from build123d import *

# Parameters (mm, degrees)
SKETCH002_R     = 2.2
SKETCH002_R_2   = 1.45
PAD002_DEPTH    = 15.5
SKETCH003_R     = 33
SKETCH003_R_2   = 2.2
PAD003_DEPTH    = 4.5
POCKET_DEPTH    = 3
POCKET001_DEPTH = 4
POCKET003_DEPTH = 2
SKETCH011_W     = 5.5
SKETCH011_H     = 11.1
POCKET004_DEPTH = 25.001
SKETCH012_W     = 3.4
SKETCH012_H     = 17.1165875376
PAD007_DEPTH    = 7.75
POCKET005_DEPTH = 229.0145930205
SKETCH017_R     = 0.75
POCKET008_DEPTH = 17.1165875376
PAD008_DEPTH    = 5
SKETCH020_R     = 0.75
POCKET009_DEPTH = 1.3324822377
FILLET_R        = 0.5
FILLET001_R     = 0.5
FILLET002_R     = 3


with BuildPart() as part:
    # Sketch002 (on Face1 of ShapeBinder) → Pad002 (new body)
    with BuildSketch(Plane.XZ.offset(37.5)):
        with BuildLine():
            Line((-32.0156211872, -8), (32.0156211872, -8))
            ThreePointArc((26.9599822671, -19.0304849165), (29.9991391555, -13.7496054463), (32.0156211872, -8))
            Line((-26.9599822671, -19.0304849165), (26.9599822671, -19.0304849165))
            ThreePointArc((-32.0156211872, -8), (-29.9991391555, -13.7496054463), (-26.9599822671, -19.0304849165))
        make_face()
        with Locations((24, -11)):
            Circle(SKETCH002_R, mode=Mode.SUBTRACT)
        with Locations((0, -11)):
            Circle(SKETCH002_R_2, mode=Mode.SUBTRACT)
        with Locations((-24, -11)):
            Circle(SKETCH002_R, mode=Mode.SUBTRACT)
    extrude(amount=PAD002_DEPTH)

    # Sketch003 (on Face9 of Pad002) → Pad003 (join)
    with BuildSketch(Plane.XZ.offset(53)):
        Circle(SKETCH003_R)
        with Locations((24, -11)):
            Circle(SKETCH003_R_2, mode=Mode.SUBTRACT)
        with Locations((-24, -11)):
            Circle(SKETCH003_R_2, mode=Mode.SUBTRACT)
    extrude(amount=PAD003_DEPTH)

    # Sketch007 (on Face2 of Pad003) → Pocket (cut)
    with BuildSketch(Plane(origin=(0, -4.5, -8), x_dir=(1, 0, 0), z_dir=(0, 0, 1))):
        with BuildLine():
            ThreePointArc((1.45, -35), (0, -33.55), (-1.45, -35))
            Line((-1.45, -35), (-1.45, -45))
            Line((-1.45, -45), (1.45, -45))
            Line((1.45, -35), (1.45, -45))
        make_face()
    extrude(amount=-POCKET_DEPTH, mode=Mode.SUBTRACT)

    # Sketch008 (on Face16 of Pocket) → Pocket001 (cut)
    with BuildSketch(Plane.XZ.offset(57.5)):
        Polygon((27.7, -13.136195996), (27.7, -8.863804004), (24, -6.727608008), (20.3, -8.863804004), (20.3, -13.136195996), (24, -15.272391992), align=None)
        Polygon((-20.3, -13.136195996), (-20.3, -8.863804004), (-24, -6.727608008), (-27.7, -8.863804004), (-27.7, -13.136195996), (-24, -15.272391992), align=None)
    extrude(amount=-POCKET001_DEPTH, mode=Mode.SUBTRACT)

    # Sketch010 (on Face10 of Pocket001) → Pocket003 (cut)
    with BuildSketch(Plane(origin=(0, -49.5, 0), x_dir=(-1, 0, 0), z_dir=(0, 1, 0))):
        with BuildLine():
            ThreePointArc((-11, -11.0000000007), (6e-10, -22), (11, -10.9999999995))
            Line((11, 0), (11, -10.9999999995))
            Line((-11, 0), (11, 0))
            Line((-11, 0), (-11, -11.0000000007))
        make_face()
    extrude(amount=-POCKET003_DEPTH, mode=Mode.SUBTRACT)

    # Sketch011 (on Face2 of Pocket003) → Pocket004 (cut, through all)
    with BuildSketch(Plane(origin=(0, -4.5, -8), x_dir=(1, 0, 0), z_dir=(0, 0, 1))):
        with Locations((17.2656211872, -40.75)):
            Rectangle(SKETCH011_W, SKETCH011_H)
    extrude(amount=-POCKET004_DEPTH, mode=Mode.SUBTRACT)

    # Sketch012 (on Face6 of Pocket004) → Pad007 (join)
    with BuildSketch(Plane(origin=(0, -53, 0), x_dir=(-1, 0, 0), z_dir=(0, 1, 0))):
        with Locations((-3.4, 23.2352590367)):
            Rectangle(SKETCH012_W, SKETCH012_H)
        with Locations((3.4, 23.2352590367)):
            Rectangle(SKETCH012_W, SKETCH012_H)
    extrude(amount=PAD007_DEPTH)

    # Sketch013 (on Face33 of Pad007) → Pocket005 (cut, through all)
    with BuildSketch(Plane(origin=(5.1, -4.5, 0), x_dir=(0, 1, 0), z_dir=(1, 0, 0))):
        with BuildLine():
            ThreePointArc((-42.925, 28.7693325629), (-44.625, 30.4693325629), (-46.325, 28.7693325629))
            Line((-46.325, 28.7693325629), (-46.325, 17.7011855106))
            ThreePointArc((-46.325, 17.7011855106), (-44.625, 16.0011855106), (-42.925, 17.7011855106))
            Line((-42.925, 28.7693325629), (-42.925, 17.7011855106))
        make_face()
    extrude(amount=-POCKET005_DEPTH, mode=Mode.SUBTRACT)

    # Sketch017 (on Face30 of Pocket005) → Pocket008 (cut)
    with BuildSketch(Plane(origin=(0, -4.5, 31.7935528056), x_dir=(1, 0, 0), z_dir=(0, 0, 1))):
        with Locations((-3.3679491924, -41.75)):
            Circle(SKETCH017_R)
        with Locations((3.3679491924, -41.75)):
            Circle(SKETCH017_R)
        with Locations((-3.3679491924, -47.5)):
            Circle(SKETCH017_R)
        with Locations((3.3679491924, -47.5)):
            Circle(SKETCH017_R)
    extrude(amount=-POCKET008_DEPTH, mode=Mode.SUBTRACT)

    # Sketch019 (on Face6 of Pocket008) → Pad008 (join)
    with BuildSketch(Plane(origin=(0, -53, 0), x_dir=(-1, 0, 0), z_dir=(0, 1, 0))):
        with BuildLine():
            ThreePointArc((29.3729634054, 15.0409115677), (29.1187588461, 15.5273269839), (28.8564999708, 16.0094475056))
            Line((25.3564999708, 16.0094475056), (28.8564999708, 16.0094475056))
            Line((25.3564999708, 16.0094475056), (25.3564999708, 14.6769652679))
            Line((25.3564999708, 14.6769652679), (29.1504409553, 14.6769652679))
            ThreePointArc((29.1504409553, 14.6769652679), (29.3637325104, 14.796555481), (29.3729634054, 15.0409115677))
        make_face()
    pad008 = extrude(amount=PAD008_DEPTH)

    # Sketch020 (on Face30 of Pad008) → Pocket009 (cut)
    with BuildSketch(Plane(origin=(0, -4.5, 16.0094475056), x_dir=(1, 0, 0), z_dir=(0, 0, 1))):
        with Locations((-27.8564999708, -44.9285714286)):
            Circle(SKETCH020_R)
        with Locations((-26.3564999708, -47.0714285714)):
            Circle(SKETCH020_R)
    pocket009 = extrude(amount=-POCKET009_DEPTH, mode=Mode.SUBTRACT)

    # Mirrored: Pad008 across Sketch019 V_Axis
    add(pad008.mirror(Plane(origin=(0, -53, 0), x_dir=(0, 1, 0), z_dir=(-1, 0, 0))))

    # Mirrored001: Pocket009 across Sketch020 V_Axis
    add(pocket009.mirror(Plane(origin=(0, -4.5, 16.0094475056), x_dir=(0, 0, 1), z_dir=(1, 0, 0))), mode=Mode.SUBTRACT)

    # Fillet
    fillet_edges = [part.edges().sort_by_distance(p)[0] for p in [
        (-5.1, -53, 23.235259),
        (-1.7, -53, 23.235259),
        (1.7, -53, 23.235259),
        (5.1, -53, 23.235259),
    ]]
    fillet(fillet_edges, radius=FILLET_R)

    # Fillet001
    fillet001_edges = [part.edges().sort_by_distance(p)[0] for p in [
        (-3.4, -45.25, 14.676965),
        (3.4, -45.25, 14.676965),
        (-3.4, -45.25, 31.793553),
        (3.4, -45.25, 31.793553),
    ]]
    fillet(fillet001_edges, radius=FILLET001_R)

    # Fillet002
    fillet002_edges = [part.edges().sort_by_distance(p)[0] for p in [
        (-25.3565, -53, 15.343206),
        (25.3565, -53, 15.343206),
    ]]
    fillet(fillet002_edges, radius=FILLET002_R)


solid = part.part
Model file for the job. Use its own axes, mm. A direction names the side the tool comes from. Give positions to 0.01 mm unless a question says otherwise; leave off trailing zeros. Loops run counter-clockwise (first coordinate to the right, second up) from the corner with the lowest first, then second, coordinate; pieces in that order, holes last. Notation, with made-up numbers: (-13, 75) - (39, 75) arc R6 cw to (39, 86) - close; hole circle Ø3 at (45.25, 42.5). An arc over 180 degrees is marked (long way). Use one line per item in the form item = value.
(1) Pull direction X, two halves, no side cores. Call faces 1 (the face through (-26.519, -52.304, 15.353)), 2 (the face through (-3.38, -49.09, 30.47)): pulls with the +X half, pulls with the -X half, needs draft (parallel to the pull), parting line crosses it, or undercut.
Determined:
face_1 = undercut
face_2 = needs draft
(2) Cut at C-C (z = 0). Give the cut face in (x, y).
Determined:
outline = (-33, -57.5) - (33, -57.5) - (33, -53) - (-33, -53) - close
(3) Drill centre lines: L1, parallel to X at y = -46.25, z = 21; L2, parallel to Z at x = 0, y = -52.3; L3, parallel to Y at x = 16.5, z = -14.5. Where is each one in solid material? Low to high.
Determined:
L1 = -5.1 to -4.12, -2.62 to -1.7, 1.7 to 2.62, 4.12 to 5.1
L2 = -19.03 to -12.45, -9.55 to -8
L3 = -57.5 to -50.8, -39.7 to -37.5
(4) Drop flat-ended pins along their axis: P1, Ø4.5, axis at y = -55.5, z = -10.5, coming from the +X side; P2, Ø5, axis at x = 8.5, y = -52, coming from the +Z side; P3, Ø1.1, axis at y = -49, z = 15.5, coming from the -X side. Give the stop position or say it passes through.
Determined:
P1 = 31.95
P2 = 32.41
P3 = -29.4
(5) Cut at B-B (x = -15). Give the cut face in (y, z).
Determined:
outline = (-57.5, -29.39) - (-53, -29.39) - (-53, -19.03) - (-37.5, -19.03) - (-37.5, -8) - (-53, -8) - (-53, 29.39) - (-57.5, 29.39) - close
(6) 3-axis set-ups, long thin cutter, end or side, ignore diameter. For faces 3 (the face through (27, -50.5, 16.009)), 4 (the face through (-24.5, -52.1, 15.3)), 5 (the face through (22, -53.5, -13)), 6 (the face through (27.51, -50.094, 15.353)), 7 (the face through (-0.314, -43.416, -12.416)): which of +Z, -Z, +X, -X, +Y, -Y reach the whole face in a straight line?
Determined:
face_3 = +Z, +X, +Y
face_4 = +Z, +Y
face_5 = -Y
face_6 = +Z
face_7 = +Y
(7) Cut at A-A (z = 26.5). Give the cut face in (x, y) (3 decimals).
Determined:
outline = (-19.666, -57.5) - (19.666, -57.5) - (19.666, -53) - (5.6, -53) arc R0.5 cw to (5.1, -52.5) - (5.1, -50.825) - (1.7, -50.825) - (1.7, -52.5) arc R0.5 cw to (1.2, -53) - (-1.2, -53) arc R0.5 cw to (-1.7, -52.5) - (-1.7, -50.825) - (-5.1, -50.825) - (-5.1, -52.5) arc R0.5 cw to (-5.6, -53) - (-19.666, -53) - close; (-5.1, -47.425) - (-1.7, -47.425) - (-1.7, -45.25) - (-5.1, -45.25) - close; (1.7, -47.425) - (5.1, -47.425) - (5.1, -45.25) - (1.7, -45.25) - close; hole circle Ø1.5 at (-3.368, -52); hole circle Ø1.5 at (-3.368, -46.25); hole circle Ø1.5 at (3.368, -52); hole circle Ø1.5 at (3.368, -46.25)
(8) Cut at D-D (z = 8). Give the cut face in (x, y).
Determined:
outline = (-32.02, -57.5) - (32.02, -57.5) - (32.02, -53) - (-32.02, -53) - close
